from build123d import *

# Parameters (mm, degrees)
SKETCH1_R           = 6.5
BOSS_EXTRUDE1_DEPTH = 45
BOSS_EXTRUDE2_DEPTH = 5
BOSS_EXTRUDE3_DEPTH = 15
SKETCH4_R           = 7.035549302
BOSS_EXTRUDE4_DEPTH = 5
SKETCH5_R           = 3
BOSS_EXTRUDE5_DEPTH = 2


with BuildPart() as part:
    # Sketch1 → Boss-Extrude1 (new body)
    with BuildSketch(Plane(origin=(0, 0, 0), x_dir=(1, 0, 0), z_dir=(0, 1, 0))):
        with Locations(Location((0, 0, 0), (0, 0, 90))):
            Circle(SKETCH1_R)
    extrude(amount=BOSS_EXTRUDE1_DEPTH)

    # Sketch2 → Boss-Extrude2 (add)
    with BuildSketch(Plane(origin=(0, 45, 0), x_dir=(1, 0, 0), z_dir=(0, 1, 0))):
        Polygon((-6.503321941, -2.684354246), (-2.700417954, -6.496668135), (2.684354246, -6.503321941), (6.496668135, -2.700417954), (6.503321941, 2.684354246), (2.700417954, 6.496668135), (-2.684354246, 6.503321941), (-6.496668135, 2.700417954), align=None)
    extrude(amount=BOSS_EXTRUDE2_DEPTH)

    # Sketch3 → Boss-Extrude3 (add)
    with BuildSketch(Plane.XZ):
        Polygon((-2.700417954, 6.496668135), (-6.503321941, 2.684354246), (-6.496668135, -2.700417954), (-2.684354246, -6.503321941), (2.700417954, -6.496668135), (6.503321941, -2.684354246), (6.496668135, 2.700417954), (2.684354246, 6.503321941), align=None)
    extrude(amount=BOSS_EXTRUDE3_DEPTH)

    # Sketch4 → Boss-Extrude4 (add)
    with BuildSketch(Plane.XZ.offset(15)):
        with Locations(Location((0, 0, 0), (0, 0, 67.570798689))):
            Circle(SKETCH4_R)
    extrude(amount=BOSS_EXTRUDE4_DEPTH)

    # Sketch5 → Boss-Extrude5 (add, symmetric)
    with BuildSketch(Plane.XY):
        with BuildLine():
            Line((1.936491673, 50), (-1.936491673, 50))
            ThreePointArc((-1.936491673, 50), (0, 57.5), (1.936491673, 50))
        make_face()
        with Locations((0, 53.5)):
            Circle(SKETCH5_R, mode=Mode.SUBTRACT)
    extrude(amount=BOSS_EXTRUDE5_DEPTH, both=True)


solid = part.part
Can you work these out from the model? Positions are in its coordinate system, mm. A direction names the side the tool comes from. Give positions to 0.01 mm unless a question says otherwise; leave off trailing zeros. Order: outer loops, then holes, each group sorted by start corner. A loop starts at its lowest first (then second) coordinate and runs counter-clockwise, first axis right, second up. Notation, with made-up numbers: M 87.5,-34.75 L 133.5,-34.75 A14 cw 133.5,-26.75 Z; hole C 1.5,53.25 d11. An arc over 180 degrees is marked long. One line per question, with ' | ' between items.
Item 1: For faces 5 (the face through (0, 57, -2)), 6 (the face through (2.63, 45, -6.12)), 7 (the face through (-4.8, -15, 4.7)), 8 (the face through (-4.56, 47.46, -4.63)), which set-ups out of +Z, -Z, +X, -X, +Y, -Y let a thin tool reach every point of the face, with its end or its side?
Answer block:
face 5: -Z, +X, -X, +Y | face 6: -Z, +X | face 7: +Z, -X, +Y | face 8: -Z, -X, +Y
Item 2: Suppose I cut it at B-B, the plane x = -1. Write out the boundary of the cut face in (y, z), then the cut area to 3 significant figures.
Answer block:
outline: M -20,-6.96 L -15,-6.96 L -15,-6.5 L 0,-6.5 L 0,-6.42 L 45,-6.42 L 45,-6.5 L 50,-6.5 L 50,-2 L 50.67,-2 L 50.67,2 L 50,2 L 50,6.5 L 45,6.5 L 45,6.42 L 0,6.42 L 0,6.5 L -15,6.5 L -15,6.96 L -20,6.96 Z; M 56.33,-2 L 57.37,-2 L 57.37,2 L 56.33,2 Z | area: 915 mm2
Item 3: I'm going to push flat-ended pins straight in: pin 1 Ø2 at (x, z) = (2.5, -6) entering from +Y; pin 2 Ø5 at (y, z) = (45.5, 1) entering from -X; pin 3 Ø6 at (x, y) = (2, 12.5) entering from -Z. Where does each tip first touch, or does it pass through?
Answer block:
pin 1: stops at y = 50 | pin 2: stops at x = -6.5 | pin 3: stops at z = -6.5
Item 4: We'd pull the mould along Y, two halves only. Please class faces 1 (the face through (4.63, 47.46, -4.56)), 2 (the face through (-6.2, 0, 2.5)), 3 (the face through (-4.7, -15, -4.9)), 4 (the face through (-6.2, 45, 2.5)): released by +Y, released by -Y, zero draft, split by the parting line, or undercut.
Answer block:
face 1: zero draft | face 2: undercut | face 3: released by +Y | face 4: undercut
Item 5: Suppose I cut it at C-C, the plane y = -3.5. Write out the boundary of the cut face in (x, z).
Answer block:
outline: M -6.5,-2.7 L -2.68,-6.5 L 2.7,-6.5 L 6.5,-2.68 L 6.5,2.7 L 2.68,6.5 L -2.7,6.5 L -6.5,2.68 Z
Item 6: Suppose I cut it at D-D, the plane z = -5.25. Write out the boundary of the cut face in (x, y), then the cut area to 3 significant figures.
Answer block:
outline: M -4.68,-20 L 4.68,-20 L 4.68,-15 L 3.94,-15 L 3.94,0 L 3.83,0 L 3.83,45 L 3.94,45 L 3.94,50 L -3.94,50 L -3.94,45 L -3.83,45 L -3.83,0 L -3.94,0 L -3.94,-15 L -4.68,-15 Z | area: 549 mm2
Item 7: Suppose I cut it at A-A, the plane y = 53.5. Write out the boundary of the cut face in (x, z).
Answer block:
outline: M -4,-2 L -3,-2 L -3,2 L -4,2 Z; M 3,-2 L 4,-2 L 4,2 L 3,2 Z
Item 8: Please list where these lines run through material, in increasing order: L1, parallel to Y at x = -1, z = 3; L2, parallel to Y at x = 2.75, z = 1.75; L3, parallel to X at y = -12, z = 2.5.
Answer block:
L1: y = -20 to 50 | L2: y = -20 to 50, 50.6 to 52.3, 54.7 to 56.4 | L3: x = -6.5 to 6.5
